from build123d import *

# Parameters (mm, degrees)
BOSS_EXTRUDE2_DEPTH = 3
SKETCH3_R           = 2
CUT_EXTRUDE1_DEPTH  = 86.498243834
SKETCH5_R           = 3.3
CUT_EXTRUDE3_DEPTH  = 2


with BuildPart() as part:
    # Sketch2 → Boss-Extrude2 (new body)
    with BuildSketch(Plane(origin=(0, 0, 0), x_dir=(1, 0, 0), z_dir=(0, 1, 0))):
        with BuildLine():
            Line((-19.525, -40.436571109), (-48, -40.436571109))
            ThreePointArc((-48, -40.436571109), (-50.952558363, -29.417473287), (-59.019097822, -21.350933827))
            Line((-59.019097822, -21.350933827), (-44.781597822, 3.309139546))
            Line((-44.781597822, 3.309139546), (-25.256597822, 37.127431563))
            Line((-25.256597822, 37.127431563), (-11.019097822, 61.787504936))
            ThreePointArc((-11.019097822, 61.787504936), (0, 58.834946573), (11.019097822, 61.787504936))
            Line((11.019097822, 61.787504936), (25.256597822, 37.127431563))
            Line((25.256597822, 37.127431563), (44.781597822, 3.309139546))
            Line((44.781597822, 3.309139546), (59.019097822, -21.350933827))
            ThreePointArc((59.019097822, -21.350933827), (50.952558363, -29.417473287), (48, -40.436571109))
            Line((48, -40.436571109), (19.525, -40.436571109))
            Line((19.525, -40.436571109), (-19.525, -40.436571109))
        make_face()
        with BuildLine():
            Line((-40.7, -37.436571109), (-40.7, -33.900672724))
            add(Edge.make_bspline(
                [(-37.7, -30.436571109), (-40.7, -30.436571109), (-40.7, -33.900672724)],
                knots=[0, 0, 0, 1.570796327, 1.570796327, 1.570796327], degree=2, weights=[1, 0.707106781, 1]))
            Line((-37.7, -30.436571109), (-34.3, -30.436571109))
            add(Edge.make_bspline(
                [(-31.3, -33.900672724), (-31.3, -30.436571109), (-34.3, -30.436571109)],
                knots=[4.71238898, 4.71238898, 4.71238898, 6.283185307, 6.283185307, 6.283185307], degree=2, weights=[1, 0.707106781, 1]))
            Line((-31.3, -33.900672724), (-31.3, -37.436571109))
            Line((-31.3, -37.436571109), (-19.525, -37.436571109))
            Line((-19.525, -37.436571109), (19.525, -37.436571109))
            Line((19.525, -37.436571109), (26.825, -37.436571109))
            Line((26.825, -37.436571109), (26.825, -33.900672724))
            add(Edge.make_bspline(
                [(29.825, -30.436571109), (26.825, -30.436571109), (26.825, -33.900672724)],
                knots=[3.141592654, 3.141592654, 3.141592654, 4.71238898, 4.71238898, 4.71238898], degree=2, weights=[1, 0.707106781, 1]))
            Line((29.825, -30.436571109), (33.225, -30.436571109))
            add(Edge.make_bspline(
                [(36.225, -33.900672724), (36.225, -30.436571109), (33.225, -30.436571109)],
                knots=[1.570796327, 1.570796327, 1.570796327, 3.141592654, 3.141592654, 3.141592654], degree=2, weights=[1, 0.707106781, 1]))
            Line((36.225, -33.900672724), (36.225, -37.436571109))
            Line((36.225, -37.436571109), (45.180375122, -37.436571109))
            ThreePointArc((45.180375122, -37.436571109), (48.354482151, -27.917473287), (55.011209172, -20.409067054))
            Line((55.011209172, -20.409067054), (52.771021611, -16.528948379))
            Line((52.771021611, -16.528948379), (49.708843785, -18.296897572))
            add(Edge.make_bspline(
                [(45.208843785, -17.430872168), (46.708843785, -20.028948379), (49.708843785, -18.296897572)],
                knots=[0, 0, 0, 1.570796327, 1.570796327, 1.570796327], degree=2, weights=[1, 0.707106781, 1]))
            Line((45.208843785, -17.430872168), (43.508843785, -14.486385795))
            add(Edge.make_bspline(
                [(45.008843785, -10.156258776), (42.008843785, -11.888309584), (43.508843785, -14.486385795)],
                knots=[4.71238898, 4.71238898, 4.71238898, 6.283185307, 6.283185307, 6.283185307], degree=2, weights=[1, 0.707106781, 1]))
            Line((45.008843785, -10.156258776), (48.071021611, -8.388309584))
            Line((48.071021611, -8.388309584), (42.183521611, 1.809139546))
            Line((42.183521611, 1.809139546), (22.658521611, 35.627431563))
            Line((22.658521611, 35.627431563), (19.008521611, 41.949417011))
            Line((19.008521611, 41.949417011), (15.946343785, 40.181467819))
            add(Edge.make_bspline(
                [(11.446343785, 41.047493222), (12.946343785, 38.449417011), (15.946343785, 40.181467819)],
                knots=[3.141592654, 3.141592654, 3.141592654, 4.71238898, 4.71238898, 4.71238898], degree=2, weights=[1, 0.707106781, 1]))
            Line((11.446343785, 41.047493222), (9.746343785, 43.991979595))
            add(Edge.make_bspline(
                [(11.246343785, 48.322106614), (8.246343785, 46.590055807), (9.746343785, 43.991979595)],
                knots=[1.570796327, 1.570796327, 1.570796327, 3.141592654, 3.141592654, 3.141592654], degree=2, weights=[1, 0.707106781, 1]))
            Line((11.246343785, 48.322106614), (14.308521611, 50.090055807))
            Line((14.308521611, 50.090055807), (9.83083405, 57.845638163))
            ThreePointArc((9.83083405, 57.845638163), (0, 55.834946573), (-9.83083405, 57.845638163))
            Line((-9.83083405, 57.845638163), (-12.071021611, 53.965519489))
            Line((-12.071021611, 53.965519489), (-9.008843785, 52.197570296))
            add(Edge.make_bspline(
                [(-7.508843785, 47.867443277), (-6.008843785, 50.465519489), (-9.008843785, 52.197570296)],
                knots=[0, 0, 0, 1.570796327, 1.570796327, 1.570796327], degree=2, weights=[1, 0.707106781, 1]))
            Line((-7.508843785, 47.867443277), (-9.208843785, 44.922956904))
            add(Edge.make_bspline(
                [(-13.708843785, 44.056931501), (-10.708843785, 42.324880693), (-9.208843785, 44.922956904)],
                knots=[4.71238898, 4.71238898, 4.71238898, 6.283185307, 6.283185307, 6.283185307], degree=2, weights=[1, 0.707106781, 1]))
            Line((-13.708843785, 44.056931501), (-16.771021611, 45.824880693))
            Line((-16.771021611, 45.824880693), (-22.658521611, 35.627431563))
            Line((-22.658521611, 35.627431563), (-42.183521611, 1.809139546))
            Line((-42.183521611, 1.809139546), (-45.833521611, -4.512845902))
            Line((-45.833521611, -4.512845902), (-42.771343785, -6.280795094))
            add(Edge.make_bspline(
                [(-41.271343785, -10.610922113), (-39.771343785, -8.012845902), (-42.771343785, -6.280795094)],
                knots=[3.141592654, 3.141592654, 3.141592654, 4.71238898, 4.71238898, 4.71238898], degree=2, weights=[1, 0.707106781, 1]))
            Line((-41.271343785, -10.610922113), (-42.971343785, -13.555408486))
            add(Edge.make_bspline(
                [(-47.471343785, -14.42143389), (-44.471343785, -16.153484698), (-42.971343785, -13.555408486)],
                knots=[1.570796327, 1.570796327, 1.570796327, 3.141592654, 3.141592654, 3.141592654], degree=2, weights=[1, 0.707106781, 1]))
            Line((-47.471343785, -14.42143389), (-50.533521611, -12.653484698))
            Line((-50.533521611, -12.653484698), (-55.011209172, -20.409067054))
            ThreePointArc((-55.011209172, -20.409067054), (-48.354482151, -27.917473287), (-45.180375122, -37.436571109))
            Line((-45.180375122, -37.436571109), (-40.7, -37.436571109))
        make_face(mode=Mode.SUBTRACT)
    extrude(amount=BOSS_EXTRUDE2_DEPTH)

    # Sketch3 → Cut-Extrude1 (cut, through all)
    with BuildSketch(Plane(origin=(0, 3, 0), x_dir=(1, 0, 0), z_dir=(0, 1, 0))):
        with Locations(Location((31.525, -35.436571109, 0), (0, 0, 270))):
            Circle(SKETCH3_R)
        with Locations(Location((-36, -35.452596513, 0), (0, 0, 270))):
            Circle(SKETCH3_R)
        with Locations(Location((-46.451470804, -9.5831653, 0), (0, 0, 270))):
            Circle(SKETCH3_R)
        with Locations(Location((48.70284921, -13.45061628, 0), (0, 0, 270))):
            Circle(SKETCH3_R)
        with Locations(Location((14.926470804, 45.019736409, 0), (0, 0, 270))):
            Circle(SKETCH3_R)
        with Locations(Location((-12.70284921, 48.903212793, 0), (0, 0, 270))):
            Circle(SKETCH3_R)
    extrude(amount=-CUT_EXTRUDE1_DEPTH, mode=Mode.SUBTRACT)

    # Sketch5 → Cut-Extrude3 (cut)
    with BuildSketch(Plane.XZ):
        with Locations(Location((48.70284921, 13.45061628, 0), (0, 0, 270))):
            Circle(SKETCH5_R)
        with Locations(Location((31.525, 35.436571109, 0), (0, 0, 270))):
            Circle(SKETCH5_R)
        with Locations(Location((-12.70284921, -48.903212793, 0), (0, 0, 270))):
            Circle(SKETCH5_R)
        with Locations(Location((14.926470804, -45.019736409, 0), (0, 0, 270))):
            Circle(SKETCH5_R)
        with Locations(Location((-36, 35.452596513, 0), (0, 0, 270))):
            Circle(SKETCH5_R)
        with Locations(Location((-46.451470804, 9.5831653, 0), (0, 0, 270))):
            Circle(SKETCH5_R)
    extrude(amount=-CUT_EXTRUDE3_DEPTH, mode=Mode.SUBTRACT)


solid = part.part
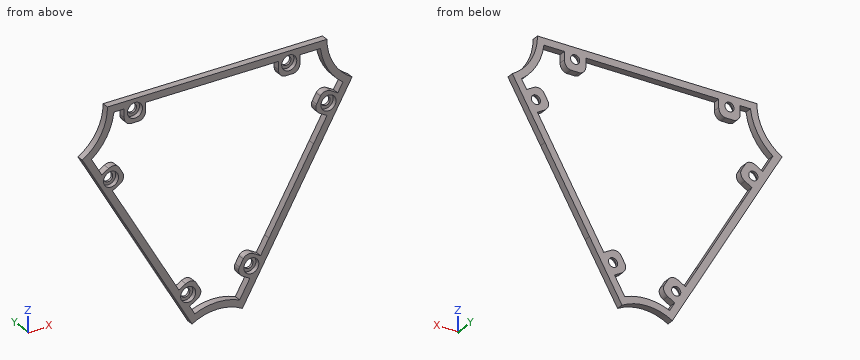
Source: CAD feature listing. Evaluate the final solid. Frame: model axes, mm. Give positions to 0.01 mm unless a question says otherwise; leave off trailing zeros. Write each loop counter-clockwise with the first axis right and the second up, starting at its lowest first coordinate (ties: lowest second). Pieces come first, ordered by that corner, then holes. Notation, with made-up numbers: M -35.5,-27.75 L 1.5,-27.75 A12 ccw 1.5,-20.75 Z; hole C 27.25,-18 d2. An arc over 180 degrees is marked long. Return JSON: item names as keys, results as strings. Group by question number.
1) First-contact query: pin 1 Ø6.5 at (x, z) = (-12.7, -48.9) entering from -Y; pin 2 Ø0.9 at (x, y) = (38.5, 1) entering from -Z. Flat tips, straight axial feed; report the tip coordinate or a pass-through.
2) Cut plane C-C, the plane y = 1.5. Give the number of separate pieces and of enclosed holes in the cut face, then the cut area to 3 significant figures.
3) Ray query, L1, parallel to X at y = 1.65, z = -41.5; L2, parallel to Z at x = 12, y = 0.1; L3, parallel to Z at x = -42, y = 1.05. Return the intervals inside material, ascending.
4) Cut plane B-B, the plane z = -21.5. Output: boundary loops of the cut face in (x, y) (3 decimals), then the cut area to 3 significant figures.
5) Cut plane A-A, the plane x = -36. Output: boundary loops of the cut face in (y, z).
Data:
{
 "1": {"pin 1": "stops at y = 2", "pin 2": "stops at z = -14.97"},
 "2": {"separate pieces": "1", "enclosed holes": "7", "area": "1,200 mm²"},
 "3": {"L1": "x = -22.73 to -19.27, 11.19 to 18.23, 19.27 to 22.73", "L2": "z = -60.09 to -54.09, -48.76 to -46.54, -43.49 to -40.38, 37.44 to 40.44", "L3": "z = -8.13 to -2.13, 6.86 to 11.87, 37.44 to 40.44"},
 "4": {"outline": "M -34.279,0 L -30.815,0 L -30.815,3 L -34.279,3 Z; M 30.815,0 L 34.279,0 L 34.279,3 L 30.815,3 Z", "area": "20.8 mm²"},
 "5": {"outline": "M 0,-18.52 L 3,-18.52 L 3,-12.52 L 0,-12.52 Z; M 0,30.44 L 3,30.44 L 3,33.45 L 2,33.45 L 2,32.15 L 0,32.15 Z; M 0,38.75 L 2,38.75 L 2,37.45 L 3,37.45 L 3,40.44 L 0,40.44 Z"}
}
